Source: CAD feature listing. Evaluate the final solid. Frame: model axes, mm. Face numbers are marked on the shaded views. A direction names the side the tool comes from. Round coordinates to 2 decimals unless told otherwise and drop trailing zeros. Order: outer loops, then holes, each group sorted by start corner. A loop starts at its lowest first (then second) coordinate and runs counter-clockwise, first axis right, second up. Notation, with made-up numbers: (74, 3.25) - (81, 3.25) arc R13 ccw to (81, 28.25) - close; hole circle Ø7 at (22.25, -16.75). An arc over 180 degrees is marked (long way). Return JSON: item names as keys, results as strings. Group by question number.
1) Access query for the marked faces 1 and 2. Directions: +Z, -Z, +X, -X, +Y, -Y. A direction counts if a zero-diameter tool reaches every point of the face in a straight line with its end or side. Return the directions, or none.
2) Section D-D, the plane z = -10. Return loops of the section in (x, y), plus the area to 3 significant figures.
3) Section C-C, the plane y = 25. Return loops of the section in (x, z), plus the area to 3 significant figures.
4) Mould query, pull axis Z, two halves, no side actions, for the marked faces 3, 4, 5 and 6. Classes: pulls with the +Z half, pulls with the -Z half, needs draft (parallel to the pull), parting line crosses it, or undercut.
5) Section B-B, the plane x = 25. Return loops of the section in (y, z), plus the area to 3 significant figures.
6) Contact query for flat-ended pins moving along their axis: P1, Ø10.5, axis at x = 21, z = 2.5, coming from the +Y side; P2, Ø8, axis at y = 23.5, z = 0, coming from the +X side. Output: stop coordinate, or through.
7) Ray query, line 1 (Y direction, x = 31, z = 15.5); line 2 (X direction, y = 2, z = 10). Return the intervals inside material, ascending. Write a range as from..to.
8) Section A-A, the plane z = 0. Return loops of the section in (x, y), plus the area to 3 significant figures.
```python
from build123d import *

# Parameters (mm, degrees)
BOSS_EXTRUDE3_DEPTH = 20
SKETCH4_R           = 2.5
CUT_EXTRUDE2_DEPTH  = 40
SKETCH5_R           = 5
CUT_EXTRUDE3_DEPTH  = 40


with BuildPart() as part:
    # Sketch1 → Boss-Extrude3 (new, symmetric)
    with BuildSketch(Plane.XY):
        with BuildLine():
            Line((0, 40), (0, 6.25))
            ThreePointArc((0, 6.25), (1.830582618, 1.830582618), (6.25, 0))
            Line((6.25, 0), (40, 0))
            Line((40, 0), (40, 5))
            Line((40, 5), (5, 5))
            Line((5, 5), (5, 40))
            Line((5, 40), (0, 40))
        make_face()
    extrude(amount=BOSS_EXTRUDE3_DEPTH, both=True)

    # Sketch4 → Cut-Extrude2 (cut)
    with BuildSketch(Plane(origin=(0, 5, 0), x_dir=(1, 0, 0), z_dir=(0, 1, 0))):
        with Locations(Location((25, -10, 0), (0, 0, 270))):
            Circle(SKETCH4_R)
        with Locations(Location((25, 10, 0), (0, 0, 270))):
            Circle(SKETCH4_R)
    extrude(amount=-CUT_EXTRUDE2_DEPTH, mode=Mode.SUBTRACT)

    # Sketch5 → Cut-Extrude3 (cut)
    with BuildSketch(Plane(origin=(5, 0, 0), x_dir=(0, 0, -1), z_dir=(1, 0, 0))):
        with Locations((0, 25)):
            Circle(SKETCH5_R)
    extrude(amount=-CUT_EXTRUDE3_DEPTH, mode=Mode.SUBTRACT)


solid = part.part
```
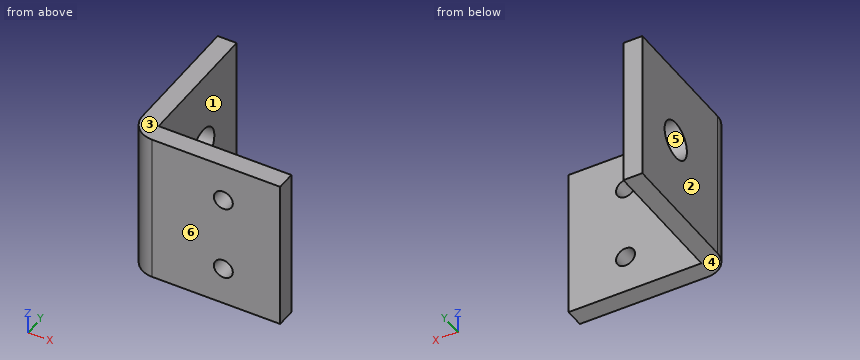
Geometry check:
{
 "1": {"face 1": "+Z, -Z, +X, +Y", "face 2": "+Z, -Z, -X, +Y, -Y"},
 "2": {"outline": "(0, 6.25) arc R6.25 ccw to (6.25, 0) - (22.5, 0) - (22.5, 5) - (5, 5) - (5, 40) - (0, 40) - close; (27.5, 0) - (40, 0) - (40, 5) - (27.5, 5) - close", "area": "342 mm2"},
 "3": {"outline": "(0, -20) - (5, -20) - (5, -5) - (0, -5) - close; (0, 5) - (5, 5) - (5, 20) - (0, 20) - close", "area": "150 mm2"},
 "4": {"face 3": "pulls with the +Z half", "face 4": "pulls with the -Z half", "face 5": "undercut", "face 6": "needs draft"},
 "5": {"outline": "(0, -20) - (5, -20) - (5, -12.5) - (0, -12.5) - close; (0, -7.5) - (5, -7.5) - (5, 7.5) - (0, 7.5) - close; (0, 12.5) - (5, 12.5) - (5, 20) - (0, 20) - close", "area": "150 mm2"},
 "6": {"P1": "y = 5", "P2": "x = 5"},
 "7": {"line 1": "0..5", "line 2": "1.67..22.5, 27.5..40"},
 "8": {"outline": "(0, 6.25) arc R6.25 ccw to (6.25, 0) - (40, 0) - (40, 5) - (5, 5) - (5, 20) - (0, 20) - close; (0, 30) - (5, 30) - (5, 40) - (0, 40) - close", "area": "317 mm2"}
}
